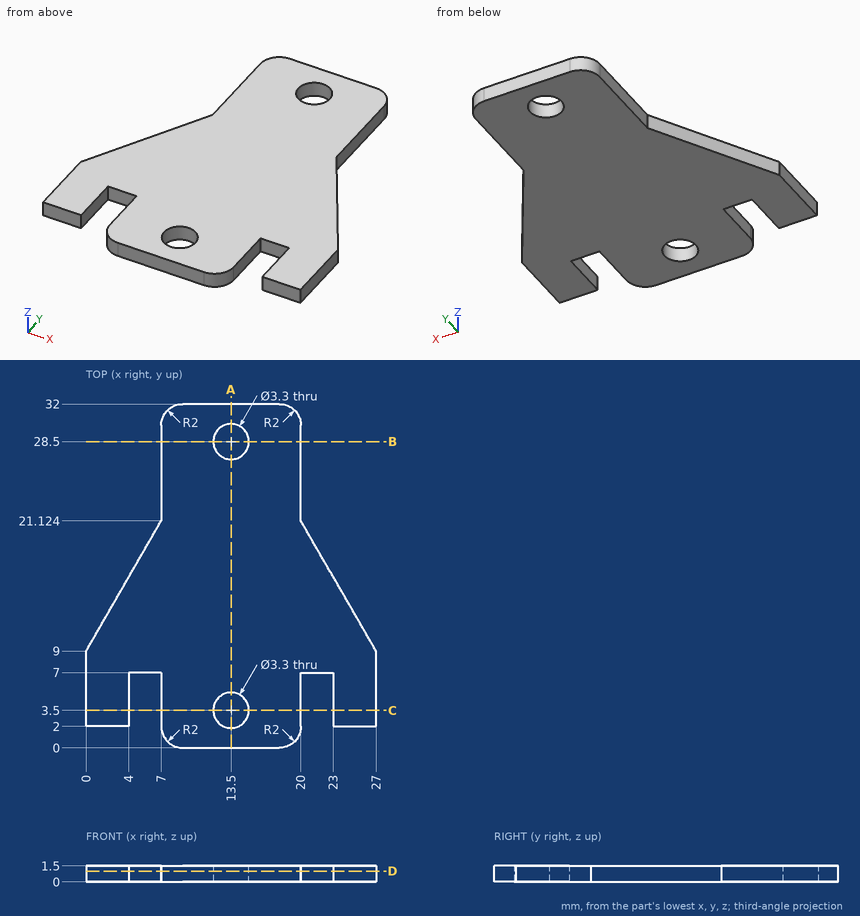
Answer from the drawing. Dimensions are ordinates in mm from the lowest x, y and z of the part. Give positions to 0.01 mm unless a question says otherwise; leave off trailing zeros. Order: outer loops, then holes, each group sorted by start corner. A loop starts at its lowest first (then second) coordinate and runs counter-clockwise, first axis right, second up. Notation, with made-up numbers: (48.25, -36.5) -> (77.25, -36.5) arc R17 ccw to (77.25, -23.5) -> close; hole circle Ø3 at (-18.5, 16). An arc over 180 degrees is marked (long way). One line per item, written item: value.
Item 1: Find section D-D, the plane z = 1. State how many separate pieces and enclosed holes the cut face has, plus the area to 3 significant figures.
Answer sheet:
separate pieces: 1
enclosed holes: 2
area: 548 mm²
Item 2: Flat-ended cylindrical pins translate along their axes: P1, Ø3, axis at x = 13.5, y = 3.5, coming from the -Z side; P2, Ø0.8, axis at x = 1, z = 1, coming from the -Y side; P3, Ø0.8, axis at y = 23.5, z = 1, coming from the -X side. Find the tip coordinate at first contact, or state that the pin passes through.
Answer sheet:
P1: through
P2: y = 2
P3: x = 7
Item 3: Find section A-A, the plane x = 13.5. Give the vertices of the cut face in (y, z), plus the area to 3 significant figures.
Answer sheet:
outline: (0, 0) -> (1.85, 0) -> (1.85, 1.5) -> (0, 1.5) -> close; (5.15, 0) -> (26.85, 0) -> (26.85, 1.5) -> (5.15, 1.5) -> close; (30.15, 0) -> (32, 0) -> (32, 1.5) -> (30.15, 1.5) -> close
area: 38.1 mm²
Item 4: Find section B-B, the plane y = 28.5. Give the vertices of the cut face in (x, z).
Answer sheet:
outline: (7, 0) -> (11.85, 0) -> (11.85, 1.5) -> (7, 1.5) -> close; (15.15, 0) -> (20, 0) -> (20, 1.5) -> (15.15, 1.5) -> close
Item 5: Straight lines are drawn through the part: probe 1 along Y at (x, z) = (13.5, 0.5); probe 2 along Y at (x, z) = (12, 1.1) (1 decimal); probe 3 along X at (y, z) = (29, 0.3). For each, find the intervals that lie inside material, in ascending order.
Answer sheet:
probe 1: 0 to 1.85, 5.15 to 26.85, 30.15 to 32
probe 2: 0 to 2.8, 4.2 to 27.8, 29.2 to 32
probe 3: 7 to 11.93, 15.07 to 20
Item 6: Find section C-C, the plane y = 3.5. Give the vertices of the cut face in (x, z).
Answer sheet:
outline: (0, 0) -> (4, 0) -> (4, 1.5) -> (0, 1.5) -> close; (7, 0) -> (11.85, 0) -> (11.85, 1.5) -> (7, 1.5) -> close; (15.15, 0) -> (20, 0) -> (20, 1.5) -> (15.15, 1.5) -> close; (23, 0) -> (27, 0) -> (27, 1.5) -> (23, 1.5) -> close
